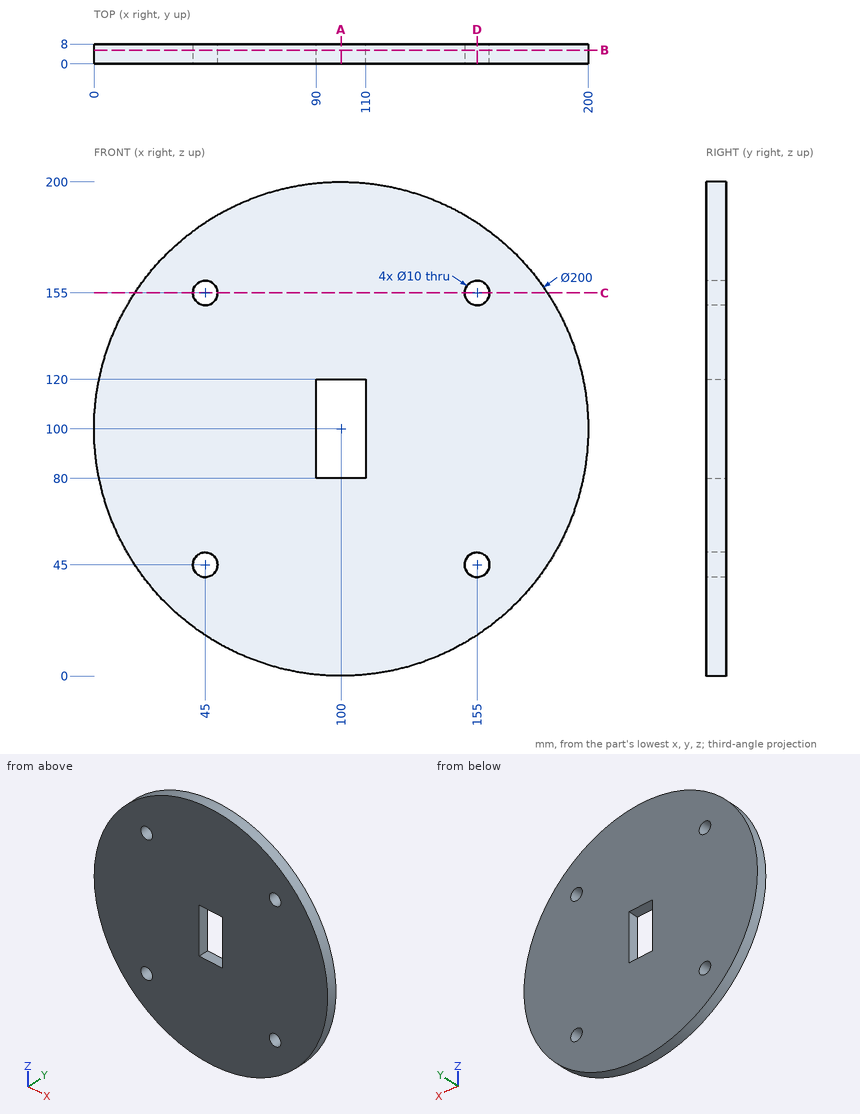
Here's the drawing with two shaded views (mm, measured from the low corner). I have some questions. Give positions to 0.01 mm unless a question says otherwise; leave off trailing zeros. Loops run counter-clockwise (first coordinate to the right, second up) from the corner with the lowest first, then second, coordinate; pieces in that order, holes last. Notation, with made-up numbers: M 21,55.25 L 30,55.25 A22 ccw 30,91.25 Z; hole C 30.25,-32 d6. An arc over 180 degrees is marked long. Use one line per item in the form item = value. Start each with the question number.
Q1. If we section it at D-D (x = 155): Write out the boundary of the cut face in (y, z), then the cut area to 3 significant figures.
Q2. If we section it at B-B (y = 5.5): Write out the boundary of the cut face in (x, z), then the cut area to 3 significant figures.
Q3. If we section it at A-A (x = 100): Write out the boundary of the cut face in (y, z), then the cut area to 3 significant figures.
Q4. If we section it at C-C (z = 155): Write out the boundary of the cut face in (x, y).
Q5. Will these pins go through, and if not, where does the flat tip stop? pin 1 Ø8 at (x, z) = (45, 155) entering from +Y; pin 2 Ø1 at (y, z) = (1, 104.5) entering from +X; pin 3 Ø4 at (x, y) = (157, 6) entering from +Z.
Q6. I need wall thicknesses on line 1 along X through (y, z) = (4, 155); line 2 along X through (y, z) = (3.25, 40.5). Which ranges of each line are inside material? Lowest first, please.
Taken from the geometry:
q1.outline = M 0,16.48 L 8,16.48 L 8,40 L 0,40 Z; M 0,50 L 8,50 L 8,150 L 0,150 Z; M 0,160 L 8,160 L 8,183.52 L 0,183.52 Z
q1.area = 1,180 mm^2
q2.outline = C 100,100 d200; hole C 45,45 d10; hole C 45,155 d10; hole M 90,80 L 110,80 L 110,120 L 90,120 Z; hole C 155,45 d10; hole C 155,155 d10
q2.area = 30,300 mm^2
q3.outline = M 0,0 L 8,0 L 8,80 L 0,80 Z; M 0,120 L 8,120 L 8,200 L 0,200 Z
q3.area = 1,280 mm^2
q4.outline = M 16.48,0 L 40,0 L 40,8 L 16.48,8 Z; M 50,0 L 150,0 L 150,8 L 50,8 Z; M 160,0 L 183.52,0 L 183.52,8 L 160,8 Z
q5.pin_1 = through
q5.pin_2 = 199.92
q5.pin_3 = 183.52
q6.line_1 = 16.48 to 40, 50 to 150, 160 to 183.52
q6.line_2 = 19.63 to 42.82, 47.18 to 152.82, 157.18 to 180.37
